The listing builds one solid part. Answer for the finished solid, in the listing's coordinates (mm). Coordinates: 2 decimals unless noted, no trailing zeros. Loops run counter-clockwise (first coordinate to the right, second up) from the corner with the lowest first, then second, coordinate; pieces in that order, holes last. Notation, with made-up numbers: (86.5, 62.25) -> (99.5, 62.25) arc R19 ccw to (99.5, 86.25) -> close; hole circle Ø5 at (-10.75, 8). An arc over 180 degrees is marked (long way). Answer in a Markdown table with one row per item.
```python
from build123d import *

# Parameters (mm, degrees)
F0_W     = 127
F0_H     = 127
F0_R     = 10.16
F0_R_2   = 12.7
F1_DEPTH = 25.4
F2_R     = 20.32
F3_SIZE  = 5.08
F5_DEPTH = 50.8964881301


with BuildPart() as f1:
    # F0 (on Front) → F1 (new body)
    with BuildSketch(Plane.XZ):
        Rectangle(F0_W, F0_H)
        with Locations((-38.1, -38.1)):
            Circle(F0_R, mode=Mode.SUBTRACT)
        with Locations((38.1, -38.1)):
            Circle(F0_R, mode=Mode.SUBTRACT)
        with Locations((-38.1, 38.1)):
            Circle(F0_R, mode=Mode.SUBTRACT)
        Circle(F0_R_2, mode=Mode.SUBTRACT)
        with Locations((38.1, 38.1)):
            Circle(F0_R, mode=Mode.SUBTRACT)
    extrude(amount=F1_DEPTH)

    # F2
    f2_edges = [f1.edges().sort_by_distance(p)[0] for p in [
        (63.5, -12.7, 63.5),
        (-63.5, -12.7, 63.5),
        (63.5, -12.7, -63.5),
        (-63.5, -12.7, -63.5),
    ]]
    fillet(f2_edges, radius=F2_R)

    # F3
    f3_edges = [f1.edges().sort_by_distance(p)[0] for p in [
        (0, 0, -63.5),
    ]]
    chamfer(f3_edges, length=F3_SIZE)

    # F4 (on face) → F5 (cut)
    with BuildSketch(Plane.XZ.offset(25.4)):
        with BuildLine():
            Line((63.5, -25.4435916758), (63.5, 25.4435916758))
            ThreePointArc((63.5, 25.4435916758), (38.0564083242, 0), (63.5, -25.4435916758))
        make_face()
    extrude(amount=-F5_DEPTH, mode=Mode.SUBTRACT)


solid = f1.part
```
Item 1: Find the intervals of material crossed by probe 1 along Z at (x, y) = (0, -8.5); probe 2 along Z at (x, y) = (-38.1, -7.75); probe 3 along Z at (x, y) = (41, -4), in increasing order.
Findings below:
| item | result |
|---|---|
| probe 1 | z = -63.5 to -12.7, 12.7 to 63.5 |
| probe 2 | z = -63.5 to -48.26, -27.94 to 27.94, 48.26 to 63.5 |
| probe 3 | z = -62.42 to -47.84, -28.36 to -11.88, 11.88 to 28.36, 47.84 to 62.42 |
Item 2: A cutting plane is placed at B-B, the plane z = -38.1. Determine the outline of the cut face in (x, y), plus the area to 3 significant figures.
Findings below:
| item | result |
|---|---|
| outline | (-63.5, -25.4) -> (-48.26, -25.4) -> (-48.26, 0) -> (-58.42, 0) -> (-63.5, -5.08) -> close; (-27.94, -25.4) -> (27.94, -25.4) -> (27.94, 0) -> (-27.94, 0) -> close; (48.26, -25.4) -> (63.5, -25.4) -> (63.5, -5.08) -> (58.42, 0) -> (48.26, 0) -> close |
| area | 2,170 mm2 |
Item 3: A cutting plane is placed at D-D, the plane y = -10. Determine the outline of the cut face in (x, z).
Findings below:
| item | result |
|---|---|
| outline | (-63.5, -43.18) arc R20.32 ccw to (-43.18, -63.5) -> (43.18, -63.5) arc R20.32 ccw to (63.5, -43.18) -> (63.5, -25.44) arc R25.44 cw to (63.5, 25.44) -> (63.5, 43.18) arc R20.32 ccw to (43.18, 63.5) -> (-43.18, 63.5) arc R20.32 ccw to (-63.5, 43.18) -> close; hole circle Ø20.32 at (-38.1, -38.1); hole circle Ø20.32 at (-38.1, 38.1); hole circle Ø25.4 at (0, 0); hole circle Ø20.32 at (38.1, -38.1); hole circle Ø20.32 at (38.1, 38.1) |
Item 4: Determine the mould class of faces 1 (the face through (61, -2.58, 33.93)), 2 (the face through (-33.412, -12.522, 29.086)), 3 (the face through (-1, -15, -63.5)), 4 (the face through (-55.11, -1.45, -54.85)) for opening direction X: +X half, -X half, draft (parallel to the pull), parting line (faces both ways), or undercut.
Findings below:
| item | result |
|---|---|
| face 1 | +X half |
| face 2 | undercut |
| face 3 | draft |
| face 4 | -X half |
Item 5: A cutting plane is placed at A-A, the plane x = -38.1. Determine the outline of the cut face in (y, z).
Findings below:
| item | result |
|---|---|
| outline | (-25.4, -63.5) -> (-5.08, -63.5) -> (0, -58.42) -> (0, -48.26) -> (-25.4, -48.26) -> close; (-25.4, -27.94) -> (0, -27.94) -> (0, 27.94) -> (-25.4, 27.94) -> close; (-25.4, 48.26) -> (0, 48.26) -> (0, 58.42) -> (-5.08, 63.5) -> (-25.4, 63.5) -> close |
Item 6: A cutting plane is placed at C-C, the plane x = 0. Determine the outline of the cut face in (y, z).
Findings below:
| item | result |
|---|---|
| outline | (-25.4, -63.5) -> (-5.08, -63.5) -> (0, -58.42) -> (0, -12.7) -> (-25.4, -12.7) -> close; (-25.4, 12.7) -> (0, 12.7) -> (0, 58.42) -> (-5.08, 63.5) -> (-25.4, 63.5) -> close |
Item 7: Flat-ended cylindrical pins translate along their axes: pin 1 Ø10 at (x, z) = (14, 14.5) entering from +Y; pin 2 Ø1.5 at (y, z) = (-2.5, -32) entering from -X. Find the tip coordinate at first contact, or state that the pin passes through.
Findings below:
| item | result |
|---|---|
| pin 1 | stops at y = 0 |
| pin 2 | stops at x = -61.67 |
